Here's how the part is built. I have some questions about the finished solid (model axes, mm). Coordinates: 2 decimals unless noted, no trailing zeros. Loops run counter-clockwise (first coordinate to the right, second up) from the corner with the lowest first, then second, coordinate; pieces in that order, holes last. Notation, with made-up numbers: M 0.25,73.5 L 28.25,73.5 A25 ccw 28.25,92.5 Z; hole C -23,11 d7. An arc over 180 degrees is marked long. Use one line per item in the form item = value. Start each with the question number.
(1) Please list where these lines run through material, in increasing order: L1, parallel to Y at x = 40, z = 1.3; L2, parallel to Y at x = 30.5, z = 1.05; L3, parallel to Y at x = 30, z = 1.15.
(2) Imagine slicing it at D-D, the plane y = -40. Please give me the cut outline in (x, z), and give its area (3 significant figures).
(3) Will these pins go through, and if not, where does the flat tip stop? P1, Ø4, axis at x = 40, y = -40, coming from the -Z side; P2, Ø1, axis at x = 25.5, z = 2.5, coming from the -Y side; P3, Ø2.5, axis at x = 5, y = -5, coming from the +Z side.
(4) Imagine slicing it at B-B, the plane x = 40. Please give me the cut outline in (y, z), and give its area (3 significant figures).
(5) Imagine slicing it at C-C, the plane z = 1. State how many separate pieces and enclosed holes the cut face has, and give its area (3 significant figures).
(6) Imagine slicing it at A-A, the plane x = 33. Please give me the cut outline in (y, z).
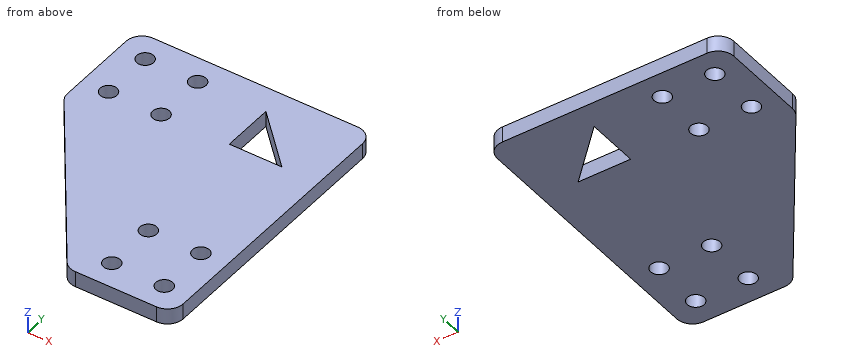
```python
from build123d import *

# Parameters (mm, degrees)
SKETCH_1_R      = 1.6
EXTRUDE_1_DEPTH = 3
FILLET_1_R      = 3


with BuildPart() as part:
    # 草图1 → 凸台-拉伸1 (new body)
    with BuildSketch(Plane.XY):
        Polygon((0, 0), (45, 0), (45, -55), (25, -55), (0, -20), align=None)
        with Locations((5, -5)):
            Circle(SKETCH_1_R, mode=Mode.SUBTRACT)
        with Locations(Location((15, -5, 0), (0, 0, 180))):
            Circle(SKETCH_1_R, mode=Mode.SUBTRACT)
        with Locations((15, -15)):
            Circle(SKETCH_1_R, mode=Mode.SUBTRACT)
        with Locations(Location((5, -15, 0), (0, 0, 180))):
            Circle(SKETCH_1_R, mode=Mode.SUBTRACT)
        with Locations((30, -50)):
            Circle(SKETCH_1_R, mode=Mode.SUBTRACT)
        with Locations(Location((40, -50, 0), (0, 0, 180))):
            Circle(SKETCH_1_R, mode=Mode.SUBTRACT)
        with Locations((40, -40)):
            Circle(SKETCH_1_R, mode=Mode.SUBTRACT)
        with Locations(Location((30, -40, 0), (0, 0, 180))):
            Circle(SKETCH_1_R, mode=Mode.SUBTRACT)
        Polygon((28, -5), (28, -15), (38, -15), align=None, mode=Mode.SUBTRACT)
    extrude(amount=EXTRUDE_1_DEPTH)

    # 圆角1
    fillet_1_edges = [part.edges().sort_by_distance(p)[0] for p in [
        (0, 0, 1.5),
        (45, 0, 1.5),
        (45, -55, 1.5),
        (25, -55, 1.5),
        (0, -20, 1.5),
    ]]
    fillet(fillet_1_edges, radius=FILLET_1_R)


solid = part.part
```
Answer:
q1.L1 = -55 to -51.6, -48.4 to -41.6, -38.4 to 0
q1.L2 = -55 to -51.52, -48.48 to -41.52, -38.48 to -15, -7.5 to 0
q1.L3 = -55 to -51.6, -48.4 to -41.6, -38.4 to -15, -7 to 0
q2.outline = M 14.29,0 L 28.4,0 L 28.4,3 L 14.29,3 Z; M 31.6,0 L 38.4,0 L 38.4,3 L 31.6,3 Z; M 41.6,0 L 45,0 L 45,3 L 41.6,3 Z
q2.area = 72.9 mm²
q3.P1 = 0
q3.P2 = -54.95
q3.P3 = through
q4.outline = M -55,0 L -51.6,0 L -51.6,3 L -55,3 Z; M -48.4,0 L -41.6,0 L -41.6,3 L -48.4,3 Z; M -38.4,0 L 0,0 L 0,3 L -38.4,3 Z
q4.area = 146 mm²
q5.separate_pieces = 1
q5.enclosed_holes = 9
q5.area = 1,920 mm²
q6.outline = M -55,0 L -15,0 L -15,3 L -55,3 Z; M -10,0 L 0,0 L 0,3 L -10,3 Z
